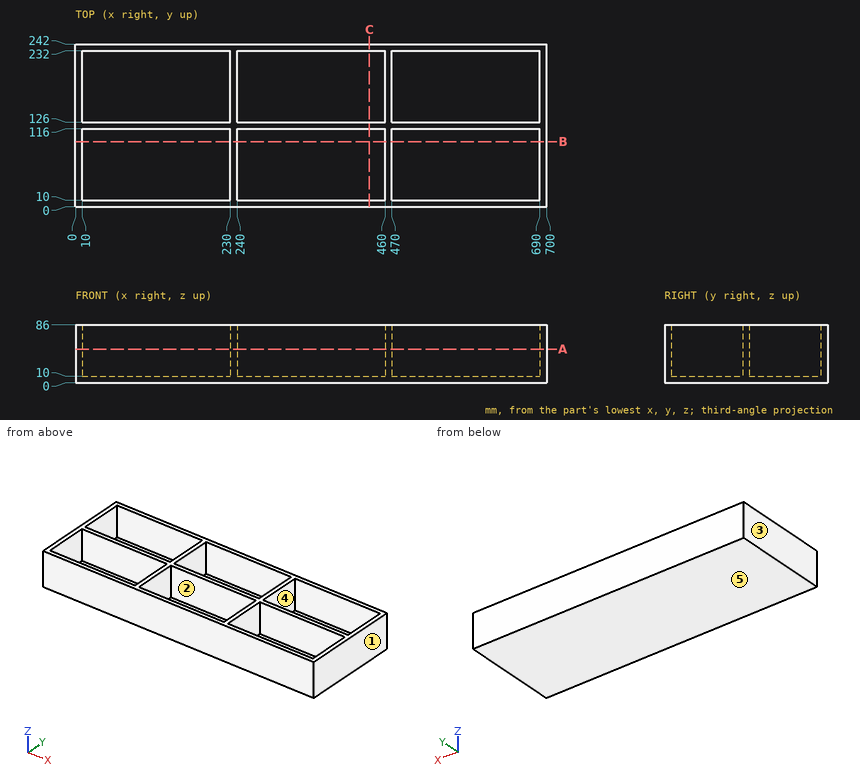
Geometry: see drawing. Coordinates: mm, zero at the bounding-box minimum. A direction names the side the tool comes from. Coordinates: 2 decimals unless noted, no trailing zeros. Write each loop counter-clockwise with the first axis right and the second up, starting at its lowest first coordinate (ties: lowest second). Pieces come first, ordered by that corner, then holes.
1) Mould query, pull axis X, two halves, no side actions, for the marked faces 1, 2 and 3. Classes: pulls with the +X half, pulls with the -X half, needs draft (parallel to the pull), parting line crosses it, or undercut.
2) Section A-A on z = 50. Output: boundary loops of the cut face in (x, y), and give its area (3 significant figures).
3) Set-up query: the marked faces 4 and 5. Return all of +Z, -Z, +X, -X, +Y, -Y with unobstructed straight access to the full face (end or side cutting, diameter ignored); none if empty.
4) Material intervals for line 1 along Y through (x, z) = (552, 68.5); line 2 along X through (y, z) = (183, 80.5); line 3 along Z through (x, y) = (666.5, 146.5), sorted ascending.
5) Pin query (flat end, axial travel): pin 1 Ø6 at (x, y) = (512.5, 152.5) entering from +Z. Return the tip coordinate at first contact, or that it passes through.
6) Section C-C on x = 436.5. Output: boundary loops of the cut face in (y, z), and give its area (3 significant figures).
7) Section B-B on y = 97. Output: boundary loops of the cut face in (x, z), and give its area (3 significant figures).
Check result:
1. face 1: pulls with the +X half
1. face 2: undercut
1. face 3: pulls with the -X half
2. outline: (0, 0) - (700, 0) - (700, 242) - (0, 242) - close; hole (10, 10) - (230, 10) - (230, 116) - (10, 116) - close; hole (10, 126) - (230, 126) - (230, 232) - (10, 232) - close; hole (240, 10) - (460, 10) - (460, 116) - (240, 116) - close; hole (240, 126) - (460, 126) - (460, 232) - (240, 232) - close; hole (470, 10) - (690, 10) - (690, 116) - (470, 116) - close; hole (470, 126) - (690, 126) - (690, 232) - (470, 232) - close
2. area: 29,500 mm2
3. face 4: +Z
3. face 5: -Z, +X, -X, +Y, -Y
4. line 1: y = 0 to 10, 116 to 126, 232 to 242
4. line 2: x = 0 to 10, 230 to 240, 460 to 470, 690 to 700
4. line 3: z = 0 to 10
5. pin 1: stops at z = 10
6. outline: (0, 0) - (242, 0) - (242, 86) - (232, 86) - (232, 10) - (126, 10) - (126, 86) - (116, 86) - (116, 10) - (10, 10) - (10, 86) - (0, 86) - close
6. area: 4,700 mm2
7. outline: (0, 0) - (700, 0) - (700, 86) - (690, 86) - (690, 10) - (470, 10) - (470, 86) - (460, 86) - (460, 10) - (240, 10) - (240, 86) - (230, 86) - (230, 10) - (10, 10) - (10, 86) - (0, 86) - close
7. area: 10,000 mm2
